For this review, take the finished solid that the model builds, in its own axes (mm). Coordinates: 2 decimals unless noted, no trailing zeros. Write each loop counter-clockwise with the first axis right and the second up, starting at its lowest first coordinate (ties: lowest second). Pieces come first, ordered by that corner, then holes.
```python
from build123d import *

# Parameters (mm, degrees)
F1_DEPTH  = 101.6
F1_FACE_W = 109.95227
F1_FACE_H = 101.6
F2_DEPTH  = 12.7


with BuildPart() as f1:
    # F0 (on Front) → F1 (new body)
    with BuildSketch(Plane.XZ):
        with BuildLine():
            Line((-60.370058, 0), (49.582213, 0))
            ThreePointArc((49.582213, 0), (-5.393922, 39.476916), (-60.370058, 0))
        make_face()
    extrude(amount=F1_DEPTH)

    # F1_face (on face) → F2 (join)
    with BuildSketch(Plane(origin=(-5.393922, -50.8, 0), x_dir=(1, 0, 0), z_dir=(0, 0, -1))):
        Rectangle(F1_FACE_W, F1_FACE_H)
    extrude(amount=F2_DEPTH)


solid = f1.part
```
Q1. Add section B-B (z = 3.5). State the section outline as (x, y) points.
Ans:
outline: (-59.06, -101.6) - (48.27, -101.6) - (48.27, 0) - (-59.06, 0) - close
Q2. Add section C-C (x = -36.5). State the section outline as (y, z) points, then the cut area to 3 significant figures.
Ans:
outline: (-101.6, -12.7) - (0, -12.7) - (0, 30.43) - (-101.6, 30.43) - close
area: 4,380 mm2
Q3. Clearance check with flat-ended pins moving along their axes: pin 1 Ø1 at (x, y) = (4.5, -31) entering from +Z; pin 2 Ø5 at (y, z) = (-51.5, 12) entering from -X; pin 3 Ø3 at (y, z) = (-27, 25.5) entering from +X. State where each tip first meets the part, or that it passes through.
Ans:
pin 1: stops at z = 38.71
pin 2: stops at x = -56.19
pin 3: stops at x = 34.06
Q4. For probe 1 along Z at (x, y) = (-4.5, -42); probe 2 along X at (y, z) = (-74, 32.5); probe 3 along Z at (x, y) = (-43, -61), list the stretches that pass through material, from the lowest coordinate up.
Ans:
probe 1: z = -12.7 to 39.47
probe 2: x = -32.98 to 22.19
probe 3: z = -12.7 to 25.64
